The model under review builds one solid part; all positions refer to its coordinate system, in mm. Face numbers are marked on the shaded views. Round coordinates to 2 decimals unless told otherwise and drop trailing zeros. Loops run counter-clockwise (first coordinate to the right, second up) from the corner with the lowest first, then second, coordinate; pieces in that order, holes last. Notation, with made-up numbers: M 68,59 L 104,59 A24 ccw 104,83 Z; hole C -5.5,-18 d10. An arc over 180 degrees is marked long. Return JSON: item names as keys, results as strings. Group by question number.
Q1. To check wall thickness, follow line 1 along X through (y, z) = (-8.5, 6.25); line 2 along Y through (x, z) = (1.5, 3); line 3 along Y through (x, z) = (10.5, 0.5). State the ranges of each line that lie inside material, in increasing order.
Q2. Draft analysis for pull direction X (two halves, no side actions). For the marked faces 1, 2, 3 and 4, state which applies: pulls with the +X half, pulls with the -X half, needs draft (parallel to the pull), parting line crosses it, or undercut.
Q3. Clearance check with flat-ended pins moving along their axes: pin 1 Ø4.5 at (x, y) = (12.37, -7.14) entering from +Z; pin 2 Ø1 at (y, z) = (10, 2) entering from +X; pin 3 Ø2 at (x, z) = (-11.5, 2) entering from +Y; pin 4 Ø1.5 at (x, z) = (-14, 5) entering from +Y. State where each tip first meets the part, or that it passes through.
Q4. Consider section A-A (y = -1.5). State the section outline as (x, z) points, and give its area (3 significant figures).
Q5. Consider section C-C (z = 1.5). State the section outline as (x, y) points.
Q6. Consider section B-B (x = -0.5). State the section outline as (y, z) points, and give its area (3 significant figures).
Q7. Consider section D-D (y = 3). State the section outline as (x, z) points, and give its area (3 significant figures).
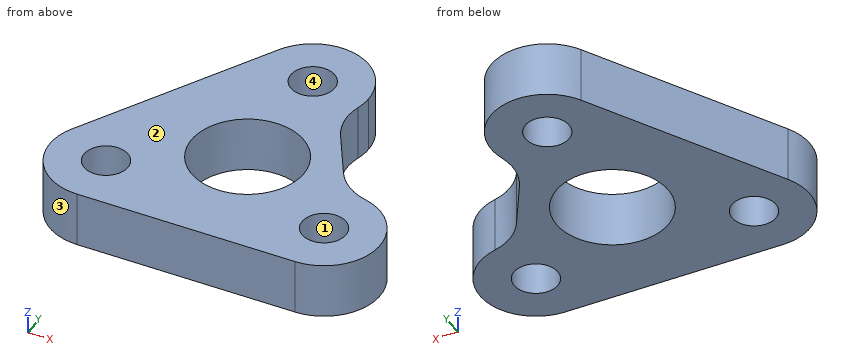
from build123d import *

# Parameters (mm, degrees)
SKETCH1_R           = 6.35
SKETCH1_R_2         = 2.4892
BOSS_EXTRUDE1_DEPTH = 6.35
FILLET1_R           = 6.35
CUT_EXTRUDE1_DEPTH  = 29.579578207
FILLET2_R           = 6.35


with BuildPart() as part:
    # Sketch1 → Boss-Extrude1 (new body)
    with BuildSketch(Plane.XY):
        Polygon((0, 26.9875), (23.371860585, -13.49375), (-23.371860585, -13.49375), align=None)
        Circle(SKETCH1_R, mode=Mode.SUBTRACT)
        with Locations((0, 14.2875)):
            Circle(SKETCH1_R_2, mode=Mode.SUBTRACT)
        with Locations((12.373337957, -7.14375)):
            Circle(SKETCH1_R_2, mode=Mode.SUBTRACT)
        with Locations((-12.373337957, -7.14375)):
            Circle(SKETCH1_R_2, mode=Mode.SUBTRACT)
    extrude(amount=BOSS_EXTRUDE1_DEPTH)

    # Fillet1
    fillet1_edges = [part.edges().sort_by_distance(p)[0] for p in [
        (0, 26.9875, 3.175),
        (23.371860585, -13.49375, 3.175),
        (-23.371860585, -13.49375, 3.175),
    ]]
    fillet(fillet1_edges, radius=FILLET1_R)

    # Sketch2 → Cut-Extrude1 (cut, through all)
    with BuildSketch(Plane.XY.offset(6.35)):
        with BuildLine():
            ThreePointArc((6.35, 14.2875), (6.00448145, 12.221416141), (5.005526767, 10.38017332))
            Line((5.005526767, 10.38017332), (11.492257175, -0.85517332))
            ThreePointArc((11.492257175, -0.85517332), (15.1582056, -1.436998542), (17.872599271, -3.96875))
            Line((17.872599271, -3.96875), (5.499261314, 17.4625))
            ThreePointArc((5.499261314, 17.4625), (6.133628997, 15.931000936), (6.35, 14.2875))
        make_face()
    extrude(amount=-CUT_EXTRUDE1_DEPTH, mode=Mode.SUBTRACT)

    # Fillet2
    fillet2_edges = [part.edges().sort_by_distance(p)[0] for p in [
        (11.492257175, -0.85517332, 3.175),
        (5.005526767, 10.38017332, 3.175),
    ]]
    fillet(fillet2_edges, radius=FILLET2_R)


solid = part.part
Values:
{
 "1": {"line 1": "x = -18.58 to -14.46, -10.29 to 10.29, 14.46 to 18.58", "line 2": "y = -13.49 to -6.17, 6.17 to 12.3, 16.27 to 20.46", "line 3": "y = -13.49 to -8.78, -5.5 to 1.08"},
 "2": {"face 1": "undercut", "face 2": "needs draft", "face 3": "pulls with the -X half", "face 4": "undercut"},
 "3": {"pin 1": "passes through", "pin 2": "stops at x = 5.93", "pin 3": "stops at y = 8.8", "pin 4": "stops at y = 4.04"},
 "4": {"outline": "M -16.45,0 L -6.17,0 L -6.17,6.35 L -16.45,6.35 Z; M 6.17,0 L 15.28,0 L 15.28,6.35 L 6.17,6.35 Z", "area": "123 mm2"},
 "5": {"outline": "M -17.87,-3.97 A6.35 ccw -12.37,-13.49 L 12.37,-13.49 A6.35 ccw 13.85,-0.97 A6.35 cw 9.82,2.03 L 6.67,7.49 A6.35 cw 6.09,12.48 A6.35 ccw -5.5,17.46 Z; hole C -12.37,-7.14 d4.98; hole C 0,0 d12.7; hole C 0,14.29 d4.98; hole C 12.37,-7.14 d4.98"},
 "6": {"outline": "M -13.49,0 L -6.33,0 L -6.33,6.35 L -13.49,6.35 Z; M 6.33,0 L 11.85,0 L 11.85,6.35 L 6.33,6.35 Z; M 16.73,0 L 20.62,0 L 20.62,6.35 L 16.73,6.35 Z", "area": "105 mm2"},
 "7": {"outline": "M -13.85,0 L -5.6,0 L -5.6,6.35 L -13.85,6.35 Z; M 5.6,0 L 9.27,0 L 9.27,6.35 L 5.6,6.35 Z", "area": "75.7 mm2"}
}
